The listing builds one solid part. Answer for the finished solid, in the listing's coordinates (mm). Coordinates: 2 decimals unless noted, no trailing zeros. Loops run counter-clockwise (first coordinate to the right, second up) from the corner with the lowest first, then second, coordinate; pieces in that order, holes last. Notation, with made-up numbers: M 26,47 L 70,47 A13 ccw 70,72 Z; hole C -6,88 d1. An arc over 180 degrees is marked long. Answer as a JSON object with one key per item and string values. Group by question number.
1. A cutting plane is placed at A-A on z = 0. Give the vertices of the cut face in (x, y).
2. Given pin 1 (1.5 mm diameter, centred on x = 15, y = 1, fed in from +Z); pin 2 (0.5 mm diameter, centred on x = 51, y = 2, fed in from +Z); pin 3 (1.1 mm diameter, centred on x = 52.5, y = 2, fed in from -Z), each flat-ended and moving along its own axis, determine where each tip first touches the part or whether it passes through.
3. A cutting plane is placed at B-B on x = 16.5. Give the vertices of the cut face in (y, z), and give its area (3 significant figures).
4. Straight lines are drawn through the part: L1, parallel to X at y = 1, z = 3; L2, parallel to Y at x = 20.5, z = 0; L3, parallel to Z at x = 23.5, y = -0.5. For each, find the intervals that lie inside material, in ascending order.
from build123d import *
from build123d.topology import SkipClean

# Parameters (mm, degrees)
SKETCH_2_R          = 3
EXTRUDE_1_DEPTH     = 4
EXTRUDE_2_DEPTH     = 2.5
SKETCH_5_R          = 2.5
EXTRUDE_3_DEPTH     = 9
MIRROR_START        = 15.5
MIRROR_1_DEPTH      = 0.381197772
MIRROR_START_2      = 15.881197772
MIRROR_1_2_DEPTH    = 4.618802228
EXTRUDE_4_DEPTH     = 5
SKETCH_10_R         = 2.5
EXTRUDE_5_DEPTH     = 6
SKETCH_11_R         = 3
EXTRUDE_6_DEPTH     = 5.5
EXTRUDE_START       = 10
SKETCH_12_R         = 3
EXTRUDE_8_DEPTH     = 10
SKETCH_13_R         = 3
EXTRUDE_9_DEPTH     = 10
SKETCH_14_OUTSIDE_W = 32.048
SKETCH_14_OUTSIDE_H = 35.048
SKETCH_14_OUTSIDE_R = 3
CUT_EXTRUDE_2_DEPTH = 59.352377883
SKETCH_15_R         = 3
EXTRUDE_10_DEPTH    = 29.5
EXTRUDE_11_DEPTH    = 26.5
CUT_EXTRUDE_START   = -3.5
SKETCH_17_W         = 2
SKETCH_17_H         = 1.2
CUT_EXTRUDE_3_DEPTH = 4
FILLET_1_R          = 0.1
SKETCH_18_R         = 3.5
EXTRUDE_12_DEPTH    = 3


with BuildPart() as part:
    # Sketch 2 → Extrude 1 (new, symmetric)
    with BuildSketch(Plane(origin=(0, 0, 0), x_dir=(0, 0, -1), z_dir=(1, 0, 0))):
        Circle(SKETCH_2_R)
    extrude_1 = extrude(amount=EXTRUDE_1_DEPTH, both=True)

    # Sketch 3 → Extrude 2 (add, symmetric)
    with BuildSketch(Plane(origin=(4, 0, 0), x_dir=(0, 0, -1), z_dir=(1, 0, 0))):
        with BuildLine():
            Line((5, 0), (5, -8))
            ThreePointArc((5, -8), (0, -13), (-5, -8))
            Line((-5, -8), (-5, 0))
            ThreePointArc((-5, 0), (0, 5), (5, 0))
        make_face()
    extrude(amount=EXTRUDE_2_DEPTH, both=True)

    # Cut-Revolve 1: read off the stored shape, not the designer's step
    # Cut-Revolve 1 outline → Cut-Revolve 1 (revolve, cut)
    with BuildSketch(Plane.YX):
        Polygon((13.0002322, 6.118936215), (4.99999958, 1.499999757), (13.0002322, 1.499999757), align=None)
    revolve(axis=Axis((0, 0, 0), (1, 0, 0)), mode=Mode.SUBTRACT)

    # Sketch 5 → Extrude 3 (add)
    with BuildSketch(Plane(origin=(6.5, 0, 0), x_dir=(0, 0, -1), z_dir=(1, 0, 0))):
        with Locations((0, -8)):
            Circle(SKETCH_5_R)
    extrude(amount=EXTRUDE_3_DEPTH)

    # Mirror 1: read off the stored shape, not the designer's step
    # Mirror 1 outline → Mirror 1 (add)
    with BuildSketch(Plane.YZ.offset(MIRROR_START)):
        with BuildLine():
            Line((-8, -5), (0, -5))
            ThreePointArc((0, -5), (5, 0), (0, 5))
            Line((0, 5), (-7.999999997, 5))
            ThreePointArc((-7.999999997, 5), (-13, 2e-09), (-8, -5))
        make_face()
    extrude(amount=MIRROR_1_DEPTH)

    # Mirror 1 2 outline → Mirror 1 2 (add)
    with BuildSketch(Plane.YZ.offset(MIRROR_START_2)):
        with BuildLine():
            Line((-8, -5), (0, -5))
            ThreePointArc((0, -5), (5, 0), (0, 5))
            Line((0, 5), (-7.999999997, 5))
            ThreePointArc((-7.999999997, 5), (-13, 2e-09), (-8, -5))
        make_face()
    extrude(amount=MIRROR_1_2_DEPTH)

    # Mirror 1 3 outline → Mirror 1 3 (revolve, cut)
    with BuildSketch(Plane.YX):
        Polygon((13.0002322, 20.500000243), (4.99999958, 20.500000243), (13.0002322, 15.881063785), align=None)
    revolve(axis=Axis((0, 0, 0), (1, 0, 0)), mode=Mode.SUBTRACT)

    # Mirror 2: Extrude 1 across plane
    add(extrude_1.mirror(Plane(origin=(11, 0, 0), x_dir=(0, 0, 1), z_dir=(1, 0, 0))))

    # Sketch 6 → Extrude 4 (add)
    with BuildSketch(Plane(origin=(26, 0, 0), x_dir=(0, 0, -1), z_dir=(1, 0, 0))):
        with BuildLine():
            Line((0, -5), (-5, -5))
            ThreePointArc((-5, -5), (-10, 0), (-5, 5))
            Line((-5, 5), (0, 5))
            ThreePointArc((0, 5), (5, 0), (0, -5))
        make_face()
    extrude_4 = extrude(amount=EXTRUDE_4_DEPTH)

    # Cut-Revolve 2: read off the stored shape, not the designer's step
    # Cut-Revolve 2 outline → Cut-Revolve 2 (revolve, cut)
    with BuildSketch(Plane.YX):
        Polygon((10.000264544, 30.195720135), (5, 26), (10.000264544, 26), align=None)
    cut_revolve_2 = revolve(axis=Axis((0, 0, 0), (1, 0, 0)), mode=Mode.SUBTRACT)

    # Sketch 10 → Extrude 5 (add)
    with BuildSketch(Plane(origin=(31, 0, 0), x_dir=(0, 0, -1), z_dir=(1, 0, 0))):
        with Locations((-5, 0)):
            Circle(SKETCH_10_R)
    extrude(amount=EXTRUDE_5_DEPTH)

    # Mirror 3: Extrude 4, Cut-Revolve 2 across plane
    add(extrude_4.mirror(Plane(origin=(34, 0, 0), x_dir=(0, 0, 1), z_dir=(1, 0, 0))))
    add(cut_revolve_2.mirror(Plane(origin=(34, 0, 0), x_dir=(0, 0, 1), z_dir=(1, 0, 0))), mode=Mode.SUBTRACT)

    # Sketch 11 → Extrude 6 (add)
    with BuildSketch(Plane(origin=(42, 0, 0), x_dir=(0, 0, -1), z_dir=(1, 0, 0))):
        Circle(SKETCH_11_R)
    extrude(amount=EXTRUDE_6_DEPTH)

    # Sketch 12 → Extrude 8 (add)
    with BuildSketch(Plane.ZY.offset(4).offset(EXTRUDE_START)):
        Circle(SKETCH_12_R)
    extrude(amount=-EXTRUDE_8_DEPTH)

    # Sketch 13 → Extrude 9 (add)
    with BuildSketch(Plane(origin=(47.5, 0, 0), x_dir=(0, 0, -1), z_dir=(1, 0, 0))):
        with Locations(Location((0, 0, 0), (0, 0, 180))):
            Circle(SKETCH_13_R)
    extrude(amount=EXTRUDE_9_DEPTH)

    # Sketch 14 outside → Cut-Extrude 2 (cut, through all)
    with SkipClean():  # the faces are left unmerged after this step: merging them gives an invalid solid
        with BuildSketch(Plane.ZY.offset(-1.5)):
            with Locations((2.5, -4)):
                Rectangle(SKETCH_14_OUTSIDE_W, SKETCH_14_OUTSIDE_H)
            Circle(SKETCH_14_OUTSIDE_R, mode=Mode.SUBTRACT)
        extrude(amount=-CUT_EXTRUDE_2_DEPTH, mode=Mode.SUBTRACT)


with BuildPart() as cut_extrude_2_piece_1:
    # of the separate pieces the step leaves, piece 1, a body of its own (cut_extrude_2_pieces)
    add(part.part.solids().sort_by_distance((37, -1.139901312, 2.775))[0])



with BuildPart() as cut_extrude_2_piece_2:
    # of the separate pieces the step leaves, piece 2, a body of its own (cut_extrude_2_pieces)
    add(part.part.solids().sort_by_distance((6.5, 0, 3))[0])


with BuildPart() as cut_extrude_2_piece_1_1:
    with SkipClean():  # the faces are left unmerged after this step: merging them gives an invalid solid
        add(cut_extrude_2_piece_1.part)

        add(cut_extrude_2_piece_2.part)  # Extrude 10 merges Cut-Extrude 2 piece 2
        # Sketch 15 → Extrude 10 (add)
        with BuildSketch(Plane.ZY.offset(-15.5)):
            Circle(SKETCH_15_R)
        extrude(amount=EXTRUDE_10_DEPTH)

    # Sketch 16 → Extrude 11 (add)
    with BuildSketch(Plane(origin=(31, 0, 0), x_dir=(0, 0, -1), z_dir=(1, 0, 0))):
        with BuildLine():
            ThreePointArc((-2.775, -1.139901312), (-2.5, 0), (-2.775, 1.139901312))
            ThreePointArc((-2.775, 1.139901312), (3, 0), (-2.775, -1.139901312))
        make_face()
    extrude(amount=EXTRUDE_11_DEPTH)

    # Sketch 17 → Cut-Extrude 3 (cut)
    with SkipClean():  # the faces are left unmerged after this step: merging them gives an invalid solid
        with BuildSketch(Plane.ZY.offset(14).offset(CUT_EXTRUDE_START)):
            with Locations((0, 2.4)):
                Rectangle(SKETCH_17_W, SKETCH_17_H)
        cut_extrude_3 = extrude(amount=-CUT_EXTRUDE_3_DEPTH, mode=Mode.SUBTRACT)

    # Fillet 1
    fillet_1_edges = [cut_extrude_2_piece_1_1.edges().sort_by_distance(p)[0] for p in [
        (-8.5, 1.8, 1),
        (-8.5, 1.8, -1),
    ]]
    fillet(fillet_1_edges, radius=FILLET_1_R)

    # Mirror 4: Cut-Extrude 3 across plane
    with SkipClean():  # the faces are left unmerged after this step: merging them gives an invalid solid
        add(cut_extrude_3.mirror(Plane.ZY.offset(-21.75)), mode=Mode.SUBTRACT)

    # Sketch 18 → Extrude 12 (add)
    with SkipClean():  # the faces are left unmerged after this step: merging them gives an invalid solid
        with BuildSketch(Plane.ZY.offset(14)):
            Circle(SKETCH_18_R)
        extrude_12 = extrude(amount=-EXTRUDE_12_DEPTH)

    # Mirror 5: Extrude 12 across plane
    with SkipClean():  # the faces are left unmerged after this step: merging them gives an invalid solid
        add(extrude_12.mirror(Plane.ZY.offset(-21.75)))


solid = cut_extrude_2_piece_1_1.part
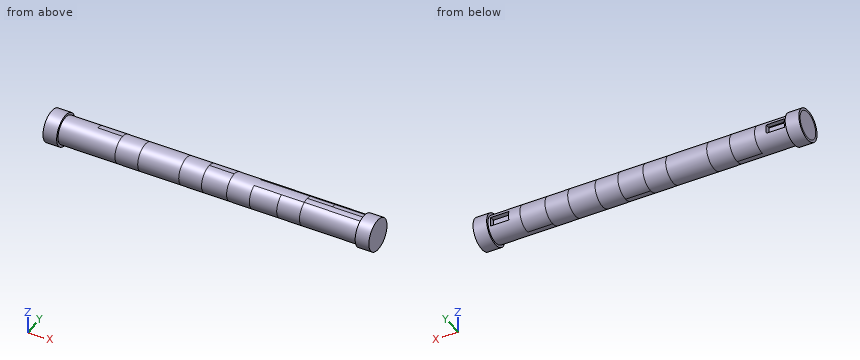
From the geometry:
{
 "1": {"outline": "M -14,-3.5 L -11,-3.5 L -11,-3 L 54.5,-3 L 54.5,-3.5 L 57.5,-3.5 L 57.5,3.5 L 54.5,3.5 L 54.5,3 L 54,3 L 54,1.8 L 50,1.8 L 50,3 L -6.5,3 L -6.5,1.8 L -10.5,1.8 L -10.5,3 L -11,3 L -11,3.5 L -14,3.5 Z"},
 "2": {"pin 1": "stops at z = 2.99", "pin 2": "stops at z = 2.44", "pin 3": "stops at z = -2.63"},
 "3": {"outline": "C 0,0 d6", "area": "28.3 mm²"},
 "4": {"L1": "x = -14 to -11, 54.5 to 57.5", "L2": "y = -3 to 3", "L3": "z = -2.96 to 2.96"}
}
